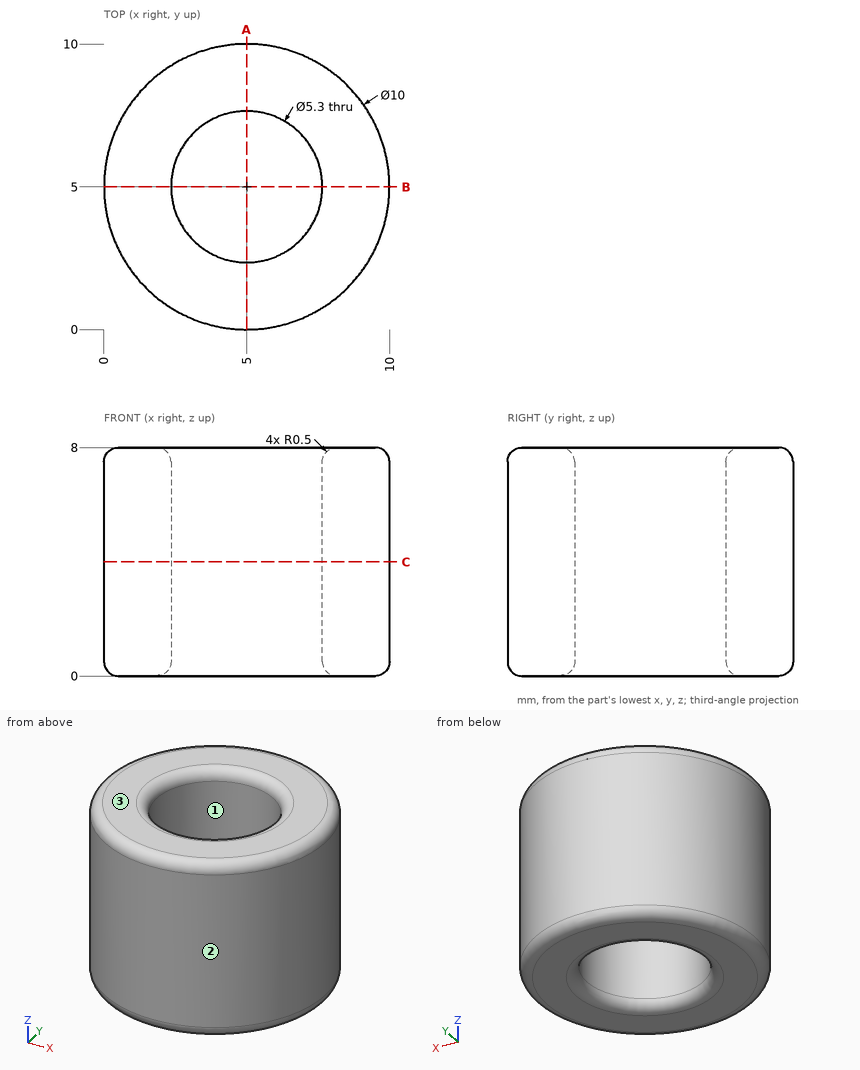
The figure shows three views and two pictorial views of one solid part (mm, origin at its lowest corner). Answer the questions. Give positions to 0.01 mm unless a question says otherwise; leave off trailing zeros. Write each loop counter-clockwise with the first axis right and the second up, starting at its lowest first coordinate (ties: lowest second). Pieces come first, ordered by that corner, then holes. Notation, with made-up numbers: (54.5, 55) - (69.5, 55) arc R21 ccw to (69.5, 76) - close; hole circle Ø9 at (-12.75, 51). An arc over 180 degrees is marked (long way). Return JSON: item names as keys, results as strings.
Q1. For a pull along Y with two mould halves and no side action, classify the marked faces 1, 2 and 3 as released by +Y, released by -Y, zero draft, split by the parting line, or undercut.
Reply:
{"face 1": "undercut", "face 2": "split by the parting line", "face 3": "zero draft"}
Q2. A cutting plane is placed at C-C, the plane z = 4. Determine the outline of the cut face in (x, y).
Reply:
{"outline": "circle Ø10 at (5, 5); hole circle Ø5.3 at (5, 5)"}
Q3. A cutting plane is placed at A-A, the plane x = 5. Determine the outline of the cut face in (y, z), and give its area (3 significant figures).
Reply:
{"outline": "(0, 0.5) arc R0.5 ccw to (0.5, 0) - (1.85, 0) arc R0.5 ccw to (2.35, 0.5) - (2.35, 7.5) arc R0.5 ccw to (1.85, 8) - (0.5, 8) arc R0.5 ccw to (0, 7.5) - close; (7.65, 0.5) arc R0.5 ccw to (8.15, 0) - (9.5, 0) arc R0.5 ccw to (10, 0.5) - (10, 7.5) arc R0.5 ccw to (9.5, 8) - (8.15, 8) arc R0.5 ccw to (7.65, 7.5) - close", "area": "37.2 mm²"}
Q4. Given P1, Ø1.5, axis at x = 6, y = 5.5, coming from the -Z side; P2, Ø1.5, axis at y = 1, z = 7, coming from the -X side, each flat-ended and moving along its own axis, determine where each tip first touches the part or whether it passes through.
Reply:
{"P1": "through", "P2": "x = 1.2"}
Q5. Consider line 1 along Y through (x, z) = (5, 5); line 2 along X through (y, z) = (4, 4.5); line 3 along X through (y, z) = (3.5, 1.5). Determine where each line is inside the solid, lowest interval first. Write a range as [from, to].
Reply:
{"line 1": "[0, 2.35], [7.65, 10]", "line 2": "[0.1, 2.55], [7.45, 9.9]", "line 3": "[0.23, 2.82], [7.18, 9.77]"}
